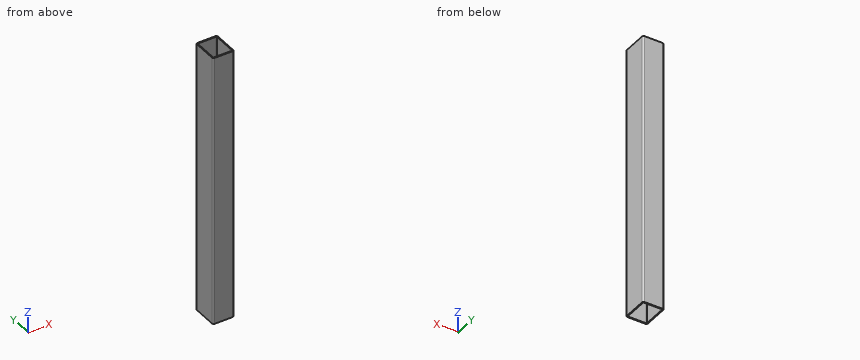
Autodesk Inventor part; units mm, degrees
ref_plane "Start plane" through (0, 0, 40) normal (0, 0, 1) x (1, 0, 0)
ref_plane "End plane" through (0, 0, 560) normal (0, 0, 1) x (1, 0, 0)
ref_plane "Work Plane4" through (-27, -475, 560) normal (0, 0, 1) x (1, 0, 0)
ref_plane "Start plane" through (0, 0, 40) normal (0, 0, 1) x (1, 0, 0)
ref_plane "End plane" through (0, 0, 560) normal (0, 0, 1) x (1, 0, 0)
sketch "Sketch" plane through (0, 0, 0) normal (0, 0, 1) x (1, 0, 0)
  line L0 (-20, -22) -> (-20, 22)
  line L1 (-17, 25) -> (17, 25)
  line L2 (20, 22) -> (20, -22)
  line L3 (17, -25) -> (-17, -25)
  arc A0 (-20, -22) -> (-17, -25) centre (-17, -22) ccw
  arc A1 (-17, 25) -> (-20, 22) centre (-17, 22) ccw
  arc A2 (20, 22) -> (17, 25) centre (17, 22) ccw
  arc A3 (17, -25) -> (20, -22) centre (17, -22) ccw
  arc A4 (-17, 23) -> (-18, 22) centre (-17, 22) ccw
  line L4 (-17, 23) -> (17, 23)
  arc A5 (18, 22) -> (17, 23) centre (17, 22) ccw
  line L5 (18, 22) -> (18, -22)
  arc A6 (17, -23) -> (18, -22) centre (17, -22) ccw
  line L6 (17, -23) -> (-17, -23)
  arc A7 (-18, -22) -> (-17, -23) centre (-17, -22) ccw
  line L7 (-18, -22) -> (-18, 22)
  line L8 (0, 35.8698) -> (0, -35.8698) construction
  line L9 (-28.8698, 0) -> (28.8698, 0) construction
  dimension "d7" = 3
  dimension "d10" = 50
  dimension "d11" = 40
  dimension "d12" = 2
  dimension "d15" = 25
  dimension "d16" = 20
extrude "Body" add sketch "Sketch" along normal up to surface (520 mm away) from surface at 40
sketch "Sketch3" plane through (0, 0, 0) normal (0, 0, 1) x (1, 0, 0)
  line L0 (0, 0) -> (10, 0)
ref_plane "Work Plane3" through (0, 0, 0) normal (0, -1, 0) x (1, 0, 0)
sketch "Sketch4" plane through (0, 0, 0) normal (0, -1, 0) x (1, 0, 0)
  line L0 (-2, 40) -> (12, 40)
  line L1 (-2, 560) -> (12, 560)
  dimension "d18" = 520
ref_plane "Work Plane4" through (-27, -475, 560) normal (0, 0, 1) x (1, 0, 0)
split "Split1" plane through (-27, -475, 560) removes the side toward (0, 0, 1)
ref_plane "Work Plane5" through (-390, -22, 40) normal (0, 0, -1) x (-1, 0, 0)
split "Split2" plane through (-390, -22, 40) removes the side toward (0, 0, -1)
equation "\"d7\" = G_IR"
equation "\"d10\" = G_H"
equation "\"d11\" = G_W"
equation "\"d12\" = G_T"
equation "\"d15\" = 0.5 * d10"
equation "\"d16\" = 0.5 * d11"
equation "\"d3\" = G_L"
equation "\"G_W\" = 40"
equation "\"G_H\" = 50"
equation "\"G_T\" = 2"
equation "\"G_IR\" = 3"
equation "\"G_L\" = d18"
equation "\"G_OFFSET_START\" = -40"
equation "\"G_OFFSET_END\" = -40"
equation "\"d13\" = -G_OFFSET_START"
equation "\"d14\" = G_OFFSET_END + B_L"
equation "\"B_L\" = 600"
properties part number "UNI EN 10305-5 - 50 x 40 x 2  - 520" material "Steel, Mild"
Geometry: final body of the model. Coordinates: model frame, mm. Round coordinates to 2 decimals unless told otherwise and drop trailing zeros. Loops run counter-clockwise (first coordinate to the right, second up) from the corner with the lowest first, then second, coordinate; pieces in that order, holes last.
Q1. Section B-B on z = 157.5. Return loops of the section in (x, y), plus the area to 3 significant figures.
Q2. Material intervals for L1, parallel to X at y = 1, z = 406; L2, parallel to Y at x = -15, z = 71.5, sorted ascending.
Q3. Section A-A on x = -4.5. Return loops of the section in (y, z), plus the area to 3 significant figures.
Q4. Section C-C on y = -10. Return loops of the section in (x, z), plus the area to 3 significant figures.
Evaluation:
1. outline: (-20, -22) arc R3 ccw to (-17, -25) - (17, -25) arc R3 ccw to (20, -22) - (20, 22) arc R3 ccw to (17, 25) - (-17, 25) arc R3 ccw to (-20, 22) - close; hole (-18, -22) arc R1 ccw to (-17, -23) - (17, -23) arc R1 ccw to (18, -22) - (18, 22) arc R1 ccw to (17, 23) - (-17, 23) arc R1 ccw to (-18, 22) - close
1. area: 337 mm2
2. L1: x = -20 to -18, 18 to 20
2. L2: y = -25 to -23, 23 to 25
3. outline: (-25, 40) - (-23, 40) - (-23, 560) - (-25, 560) - close; (23, 40) - (25, 40) - (25, 560) - (23, 560) - close
3. area: 2,080 mm2
4. outline: (-20, 40) - (-18, 40) - (-18, 560) - (-20, 560) - close; (18, 40) - (20, 40) - (20, 560) - (18, 560) - close
4. area: 2,080 mm2
